Verification items for the finished model (mm, model axes). Give positions to 0.01 mm unless a question says otherwise; leave off trailing zeros. Order: outer loops, then holes, each group sorted by start corner. A loop starts at its lowest first (then second) coordinate and runs counter-clockwise, first axis right, second up.
(1) Scan lines: L1, parallel to X at y = -2.25, z = -1.65; L2, parallel to X at y = -2.1, z = 2; L3, parallel to Y at x = 23, z = 2.7. Record each from-to range of solid material in increasing order.
(2) Sectioned sample at A-A on x = 20. Record the cut outline in (y, z).
(3) Gauge pin test, flat ends, axial feed: pin 1 (1.5 mm diameter, centred on x = 14, z = -1, fed in from -Y); pin 2 (1 mm diameter, centred on x = 19, y = 1.5, fed in from -Z); pin 3 (1 mm diameter, centred on x = 21, y = -2.5, fed in from +Z). Record the tip position at first contact, or that the pin passes through.
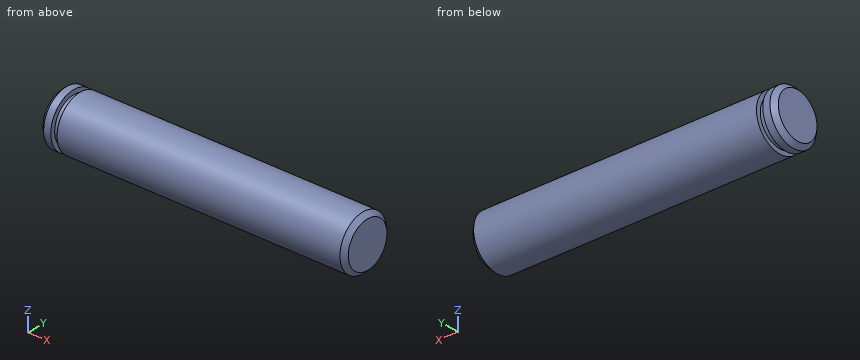
```python
from build123d import *


with BuildPart() as part:
    # Sketch1 → Revolve1 (revolve)
    with BuildSketch(Plane.XY, mode=Mode.PRIVATE) as revolve1_sk:
        Polygon((0, 0), (0, 3), (31.5, 3), (32, 2.5), (32, 0), align=None)
    revolve(revolve1_sk.sketch.rotate(Axis((32, 0, 0), (-1, 0, 0)), 270), axis=Axis((32, 0, 0), (-1, 0, 0)))

    # Sketch2 → Revolve2 (revolve)
    with BuildSketch(Plane.XY, mode=Mode.PRIVATE) as revolve2_sk:
        Polygon((-2, 0), (-2, 2.5), (-1.5, 3), (-0.7, 3), (-0.7, 2.5), (0, 2.5), (0, 0), align=None)
    revolve(revolve2_sk.sketch.rotate(Axis((0, 0, 0), (-1, 0, 0)), 270), axis=Axis((0, 0, 0), (-1, 0, 0)))


solid = part.part
```
Ans:
1. L1: x = -1.71 to -0.7, 0 to 31.71
1. L2: x = -1.6 to -0.7, 0 to 31.6
1. L3: y = -1.31 to 1.31
2. outline: circle Ø6 at (0, 0)
3. pin 1: stops at y = -2.99
3. pin 2: stops at z = -2.83
3. pin 3: stops at z = 2.24
